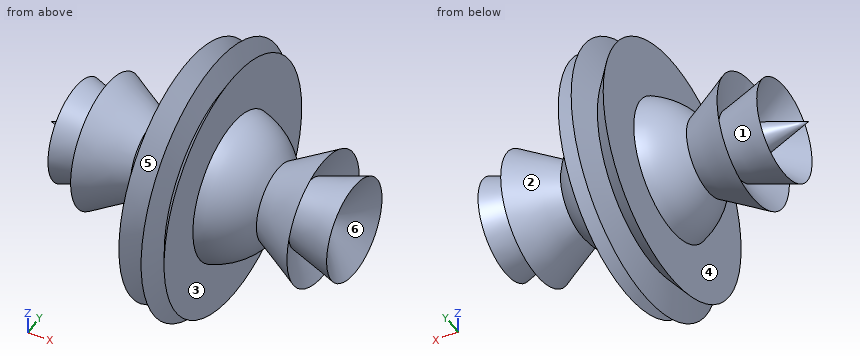
```python
from build123d import *


# Not quite as in the source:
# - a feature names something its author has since deleted; it is built from what else it names


with BuildPart() as f1:
    # F0 (on Top) → F1 (revolve)
    with BuildSketch(Plane.XY):
        with BuildLine():
            Line((37.1953770518, 22.2900286317), (21.6585689027, 13.2690012092))
            ThreePointArc((21.6585689027, 13.2690012092), (15.0259859449, 20.4787633021), (6.1581879854, 24.6421736204))
            Line((6.1581879854, 24.6421736204), (6.1581879854, 42.3834808171))
            Line((6.1581879854, 42.3834808171), (3.0790939927, 36.7608899251))
            Line((3.0790939927, 36.7608899251), (0, 45.5001890659))
            Line((0, 45.5001890659), (-3.0941891787, 34.9035797321))
            Line((-3.0941891787, 34.9035797321), (-9.3218332717, 42.48192312))
            Line((-9.3218332717, 42.48192312), (-9.3218332717, 23.6275987873))
            ThreePointArc((-9.3218332717, 23.6275987873), (-16.3331401043, 19.4522115538), (-21.6585689027, 13.2690012092))
            Line((-21.6585689027, 13.2690012092), (-37.1953770518, 22.2900286317))
            Line((-37.1953770518, 22.2900286317), (-31.91267699, 11.7950700223))
            Line((-31.91267699, 11.7950700223), (-47.922976315, 17.042549327))
            Line((-47.922976315, 17.042549327), (-36.8364676833, 6.3755996525))
            Line((-36.8364676833, 6.3755996525), (-56.2179237604, 0))
            Line((-56.2179237604, 0), (36.3256136068, 0))
            Line((36.3256136068, 0), (47.922976315, 17.042549327))
            Line((47.922976315, 17.042549327), (31.91267699, 11.7950700223))
            Line((31.91267699, 11.7950700223), (37.1953770518, 22.2900286317))
        make_face()
    revolve(axis=Axis((-9.9461550768, 0, 0), (1, 0, 0)))


solid = f1.part
```
Here's how the part is built. I have some questions about the finished solid (model axes, mm). Face numbers are marked on the shaded views. A direction names the side the tool comes from. Coordinates: 2 decimals unless noted, no trailing zeros. Order: outer loops, then holes, each group sorted by start corner. A loop starts at its lowest first (then second) coordinate and runs counter-clockwise, first axis right, second up. Notation, with made-up numbers: (46.5, -31.75) - (66.5, -31.75) arc R28 cw to (66.5, 4.25) - close; hole circle Ø10 at (54.5, -20). An arc over 180 degrees is marked (long way). One line per question, with ' | ' between items.
(1) Suppose I cut it at C-C on x = -18. List the corners of the cut face in (y, z) for me.
Report:
outline: circle Ø35.84 at (0, 0)
(2) If I drill on L1, parallel to X at y = -21.5, z = -2.5; L2, parallel to Y at x = -39.5, z = 5; L3, parallel to X at y = -41.5, z = 3.5, over which ranges is the centre line in solid material (lowest first)?
Report:
L1: x = -36.87 to -36.08, -13.29 to 13.29, 36.08 to 36.87 | L2: y = -13.38 to -7.41, -2.29 to 2.29, 7.41 to 13.38 | L3: x = -9.32 to -8.64, -1.13 to 1.36, 5.76 to 6.16
(3) Suppose I cut it at A-A on x = -33.5. List the corners of the cut face in (y, z) for me, and give its area (3 significant figures).
Report:
outline: circle Ø40.29 at (0, 0); circle Ø24.63 at (0, 0); hole circle Ø29.9 at (0, 0) | area: 1,050 mm2
(4) Will these pins go through, and if not, where does the flat tip stop? pin 1 (5 mm diameter, centred on x = -44, z = 21, fed in from -Y); pin 2 (8 mm diameter, centred on y = -17, z = -9.5, fed in from -X); pin 3 (3 mm diameter, centred on y = 8, z = 14.5, fed in from +X); pin 4 (10 mm diameter, centred on y = -12.5, z = 19.5, fed in from +X).
Report:
pin 1: passes through | pin 2: stops at x = -47.92 | pin 3: stops at x = 47.92 | pin 4: stops at x = 37.2
(5) If we mould it in two halves opening along Z, with no side actions, what happens to the marked faces 1, 2 and 3? For each: pulls with the +Z half, pulls with the -Z half, needs draft (parallel to the pull), parting line crosses it, or undercut.
Report:
face 1: undercut | face 2: parting line crosses it | face 3: needs draft
(6) For the marked faces 4, 5 and 6, which set-ups out of +Z, -Z, +X, -X, +Y, -Y let a thin tool reach every point of the face, with its end or its side?
Report:
face 4: -X | face 5: none | face 6: +X
(7) Suppose I cut it at B-B on z = 20.5. State how many separate pieces and enclosed holes the cut face has, and give its area (3 significant figures).
Report:
separate pieces: 3 | enclosed holes: 0 | area: 1,370 mm2
